Check sheet for the drawn part. Datum: minimum x, y, z corner. Units: mm. A direction names the side the tool comes from. Coordinates: 2 decimals unless noted, no trailing zeros. Order: outer loops, then holes, each group sorted by start corner. A loop starts at its lowest first (then second) coordinate and runs counter-clockwise, first axis right, second up. Notation, with made-up numbers: (7.25, -22.5) - (52.25, -22.5) arc R8 cw to (52.25, -9.5) - close; hole circle Ø2 at (-22.5, 24). An arc over 180 degrees is marked (long way). Return JSON: item names as keys, results as strings. Group by question number.
Item 1: Draft check along X on the marked faces 1, 2, 3 and 4. Enter one of: pulls with the +X half, pulls with the -X half, needs draft (parallel to the pull), parting line crosses it, or undercut.
Item 2: Tool access check on the marked faces 5, 6 and 7. Record the directions out of +Z, -Z, +X, -X, +Y, -Y that give a thin tool (end or side, any length) a straight path to the whole face; none if there is none.
Item 3: Section check B-B on x = 58.2. Enter the section's corners in (y, z) (3 decimals), then the cut area to 3 significant figures.
Item 4: Gauge pin test, flat ends, axial feed: pin 1 (4.5 mm diameter, centred on x = 81.77, y = 9.63, fed in from +Z); pin 2 (5 mm diameter, centred on x = 8.2, z = 9.5, fed in from +Y); pin 3 (10 mm diameter, centred on y = 27, z = 51.5, fed in from +X); pin 4 (5 mm diameter, centred on y = 31, z = 24, fed in from -X). Record the tip position at first contact, or that the pin passes through.
Item 5: Section check C-C on y = 24. Enter the section's corners in (x, z), then the cut area to 3 significant figures.
Item 6: Scan lines: probe 1 along X at (y, z) = (1, 9.5); probe 2 along X at (y, z) = (14, 10.5); probe 3 along X at (y, z) = (56, 57). Record each from-to range of solid material in increasing order.
Item 7: Section check D-D on z = 49.5. Enter the section's corners in (x, y).
Item 8: Section check A-A on x = 34.63. Enter the section's corners in (y, z), then the cut area to 3 significant figures.
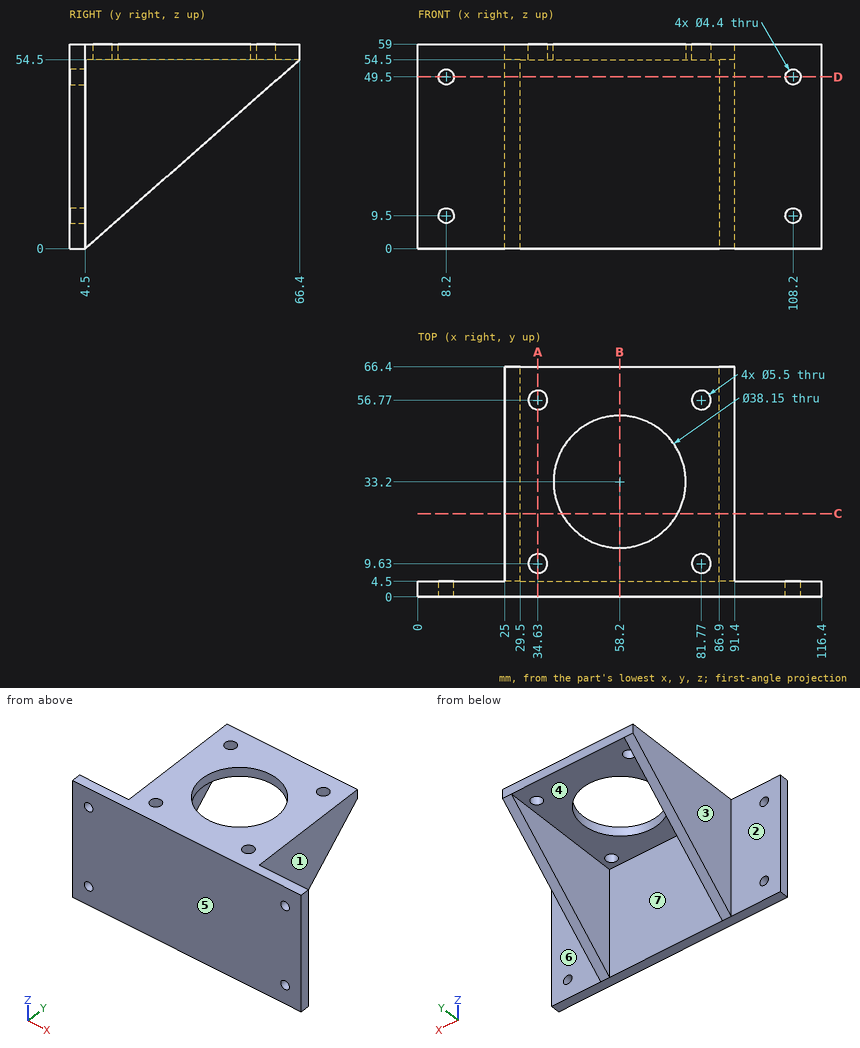
Computed:
{
 "1": {"face 1": "pulls with the +X half", "face 2": "needs draft", "face 3": "pulls with the -X half", "face 4": "undercut"},
 "2": {"face 5": "+Z, -Z, +X, -X, -Y", "face 6": "+Z, -Z, +X, +Y", "face 7": "-Z, +Y"},
 "3": {"outline": "(0, 0) - (4.5, 0) - (4.5, 54.5) - (14.125, 54.5) - (14.125, 59) - (0, 59) - close; (52.275, 54.5) - (66.4, 54.5) - (66.4, 59) - (52.275, 59) - close", "area": "372 mm²"},
 "4": {"pin 1": "passes through", "pin 2": "stops at y = 4.5", "pin 3": "stops at x = 91.4", "pin 4": "stops at x = 25"},
 "5": {"outline": "(25, 17.17) - (29.5, 17.17) - (29.5, 54.5) - (41.49, 54.5) - (41.49, 59) - (25, 59) - close; (74.91, 54.5) - (86.9, 54.5) - (86.9, 17.17) - (91.4, 17.17) - (91.4, 59) - (74.91, 59) - close", "area": "484 mm²"},
 "6": {"probe 1": "x = 0 to 6, 10.4 to 106, 110.4 to 116.4", "probe 2": "x = 25 to 29.5, 86.9 to 91.4", "probe 3": "x = 25 to 31.99, 37.27 to 79.13, 84.41 to 91.4"},
 "7": {"outline": "(0, 0) - (6, 0) - (6, 4.5) - (0, 4.5) - close; (10.4, 0) - (106, 0) - (106, 4.5) - (91.4, 4.5) - (91.4, 60.72) - (86.9, 60.72) - (86.9, 4.5) - (29.5, 4.5) - (29.5, 60.72) - (25, 60.72) - (25, 4.5) - (10.4, 4.5) - close; (110.4, 0) - (116.4, 0) - (116.4, 4.5) - (110.4, 4.5) - close"},
 "8": {"outline": "(0, 0) - (4.5, 0) - (4.5, 54.5) - (6.88, 54.5) - (6.88, 59) - (0, 59) - close; (12.38, 54.5) - (54.02, 54.5) - (54.02, 59) - (12.38, 59) - close; (59.52, 54.5) - (66.4, 54.5) - (66.4, 59) - (59.52, 59) - close", "area": "495 mm²"}
}
